For this review, take the finished solid that the model builds, in its own axes (mm). A direction names the side the tool comes from. Give positions to 0.01 mm unless a question says otherwise; leave off trailing zeros. Order: outer loops, then holes, each group sorted by start corner. A loop starts at its lowest first (then second) coordinate and runs counter-clockwise, first axis right, second up. Notation, with made-up numbers: (85.25, -28.75) - (133.25, -28.75) arc R23 cw to (133.25, -1.75) - close; hole circle Ø5 at (58, -16.75). An arc over 180 degrees is marked (long way). Use a Markdown table: item, result. Add a question column.
1) Machinability: for faces 4 (the face through (-242.37, -125.525, 1.479)), 5 (the face through (-214.32, -123.41, 1.48)), 6 (the face through (-24.751, -65.135, 1.479)), which of the approach directions +Z, -Z, +X, -X, +Y, -Y give a long, thin tool a straight path to every point of the face, cutting with its end or side? Answer none if there is none.
2) We need section C-C on y = -44.5. Write out the cut boundary in (x, z).
3) We need section B-B on z = 2.45. Give the number of separate pieces and of enclosed holes in the cut face, then the cut area to 3 significant figures.
4) Mouldability with a two-part tool opening along X and no side actions: class faces 1 (the face through (-270.05, -107.925, 1.479)), 2 (the face through (-117.616, -108.409, 1.479)), 3 (the face through (-169, -32, 3)) as released by +X, released by -X, zero draft, split by the parting line, or undercut.
5) Clearance check with flat-ended pins moving along their axes: P1, Ø1.5, axis at y = -16.5, z = 2.5, coming from the -X side; P2, Ø0.9, axis at x = -158.5, z = 2, coming from the +Y side; P3, Ø1.5, axis at y = -10.5, z = 2, coming from the -X side. State where each tip first meets the part, or that it passes through.
6) Wall thickness on L1, parallel to X at y = -106, z = 0.95; L2, parallel to X at y = -125, z = 1.9; L3, parallel to Y at x = -226.5, z = 2.65: over which ranges is each line inside the solid? List them lowest first.
7) We need section A-A on x = -33. Write out the cut boundary in (y, z), then the cut area to 3 significant figures.
```python
from build123d import *

# Parameters (mm, degrees)
BOSS_EXTRU_1_DEPTH = 3


with BuildPart() as part:
    # Esquisse1 → Boss.-Extru.1 (new body)
    with BuildSketch(Plane.XY):
        Polygon((-179.931816419, -11.401531345), (-180.017838024, -11.701531345), (-185.57619805, -31.086289447), (-167.791072806, -36.185021562), (-127.904950096, -24.747859919), (-17.351203316, 6.946262636), (-14.877374555, 5.574907028), (2.556514314, -55.224288823), (1.185265633, -57.698086926), (-51.424530344, -72.783703169), (-57.630729871, -89.716454796), (-63.024672228, -92.169507978), (-104.349665635, -118.563827288), (-107.470944884, -118.248029963), (-128.050089261, -98.290842938), (-133.151477342, -93.715936913), (-202.439042401, -93.715936913), (-207.540430482, -98.290842938), (-228.119574859, -118.248029963), (-231.240854108, -118.563827288), (-272.565847516, -92.169507978), (-277.959789872, -89.716454796), (-284.165989399, -72.783703169), (-336.775785376, -57.698086926), (-338.147034057, -55.224288823), (-320.713145188, 5.574907028), (-318.239316427, 6.946262636), (-207.685569647, -24.747859919), (-203.944682562, -11.701531345), (-203.858660957, -11.401531345), (-205.982988252, -11.401531345), (-221.327812729, -7.001473731), (-228.053301524, -5.072970852), (-324.305573392, 22.521130566), (-330.707501003, 18.97225141), (-353.72243999, -61.290379239), (-350.173829458, -67.692242105), (-294.328030452, -83.705767284), (-288.532091821, -99.519179156), (-251.042661762, -116.568594893), (-233.45174982, -134.735979634), (-226.135810249, -134.851076098), (-202.175390102, -111.650948678), (-133.415129641, -111.650948678), (-109.454709494, -134.851076098), (-102.138769923, -134.735979634), (-84.547857981, -116.568594893), (-47.058427922, -99.519179156), (-41.262489291, -83.705767284), (14.583309715, -67.692242105), (18.131920247, -61.290379239), (-4.88301874, 18.97225141), (-11.284946351, 22.521130566), (-107.537218219, -5.072970852), (-114.262707014, -7.001473731), (-123.876268292, -9.758118068), (-129.607531491, -11.401531345), (-167.175777529, -11.401531345), align=None)
        Polygon((-226.456549288, -126.726039887), (-228.072581173, -129.499661036), (-231.282623491, -129.486946945), (-232.876633924, -126.700611704), (-231.260602039, -123.926990555), (-228.050559721, -123.939704646), align=None, mode=Mode.SUBTRACT)
        Polygon((-201.720052379, -99.68218544), (-200.986265397, -102.807259839), (-203.325765724, -105.005275206), (-206.399053033, -104.078216174), (-207.132840016, -100.953141775), (-204.793339689, -98.755126408), align=None, mode=Mode.SUBTRACT)
        Polygon((-278.801584282, -92.701419409), (-279.761510176, -95.764600045), (-282.89426537, -96.464870154), (-285.067094671, -94.101959627), (-284.107168778, -91.03877899), (-280.974413583, -90.338508881), align=None, mode=Mode.SUBTRACT)
        Polygon((-341.674936445, -60.693756917), (-343.381773974, -63.412440235), (-346.589641557, -63.293617233), (-348.09067161, -60.456110913), (-346.38383408, -57.737427596), (-343.175966498, -57.856250598), align=None, mode=Mode.SUBTRACT)
        Polygon((-102.716844109, -126.851692582), (-104.440215275, -129.559925429), (-107.647299303, -129.421558643), (-109.131012166, -126.574959009), (-107.407640999, -123.866726161), (-104.200556971, -124.005092948), align=None, mode=Mode.SUBTRACT)
        Polygon((-129.102521286, -103.979530359), (-132.134816884, -105.032961295), (-134.563262635, -102.933631743), (-133.959412787, -99.780871255), (-130.927117189, -98.727440319), (-128.498671438, -100.826769871), align=None, mode=Mode.SUBTRACT)
        Polygon((-51.178552765, -91.36063702), (-50.649763202, -94.526851626), (-53.127390703, -96.567904124), (-56.133807767, -95.442742016), (-56.662597331, -92.27652741), (-54.18496983, -90.235474912), align=None, mode=Mode.SUBTRACT)
        Polygon((10.897318032, -57.794933915), (12.502351781, -60.574933915), (10.897318032, -63.354933915), (7.687250536, -63.354933915), (6.082216787, -60.574933915), (7.687250536, -57.794933915), align=None, mode=Mode.SUBTRACT)
        Polygon((-217.840116073, -13.876277124), (-214.696831686, -14.527657653), (-213.689301579, -17.575512049), (-215.825055858, -19.971985915), (-218.968340246, -19.320605385), (-219.975870353, -16.272750989), align=None, mode=Mode.SUBTRACT)
        Polygon((-326.25776259, 15.467139628), (-323.377643582, 16.884689567), (-320.709949819, 15.09920831), (-320.922375064, 11.896177113), (-323.802494072, 10.478627174), (-326.470187835, 12.264108431), align=None, mode=Mode.SUBTRACT)
        Polygon((-169.385770719, -24.817214521), (-166.175746894, -24.833958909), (-164.585236046, -27.622293282), (-166.204749024, -30.393883267), (-169.414772849, -30.37713888), (-171.005283697, -27.588804506), align=None, mode=Mode.SUBTRACT)
        Polygon((-117.981174931, -13.809459943), (-115.672169645, -16.039488624), (-116.448928491, -19.154160201), (-119.534692623, -20.038803095), (-121.84369791, -17.808774414), (-121.066939064, -14.694102838), align=None, mode=Mode.SUBTRACT)
        Polygon((-12.039253575, 16.891491339), (-9.240055353, 15.320178943), (-9.201252694, 12.110345974), (-11.961648258, 10.471825402), (-14.76084648, 12.043137798), (-14.799649138, 15.252970767), align=None, mode=Mode.SUBTRACT)
    extrude(amount=BOSS_EXTRU_1_DEPTH)


solid = part.part
```
Checked values:
| question | item | result |
|---|---|---|
| 1 | face 4 | +Z, -Z, -X, -Y |
| 1 | face 5 | +Z, -Z, -Y |
| 1 | face 6 | +Z, -Z |
| 2 | outline | (-348.91, 0) - (-335.07, 0) - (-335.07, 3) - (-348.91, 3) - close; (-0.52, 0) - (13.32, 0) - (13.32, 3) - (-0.52, 3) - close |
| 3 | separate pieces | 1 |
| 3 | enclosed holes | 13 |
| 3 | area | 11,900 mm² |
| 4 | face 1 | released by -X |
| 4 | face 2 | undercut |
| 4 | face 3 | zero draft |
| 5 | P1 | x = -341.09 |
| 5 | P2 | y = -11.4 |
| 5 | P3 | x = -339.37 |
| 6 | L1 | -274.28 to -250.91, -215.49 to -120.1, -84.68 to -61.31 |
| 6 | L2 | -242.88 to -231.89, -227.44 to -215.96, -119.63 to -108.13, -103.68 to -92.71 |
| 6 | L3 | -134.85 to -126.8, -126.65 to -116.68, -19.35 to -5.52 |
| 7 | outline | (-81.34, 0) - (-67.5, 0) - (-67.5, 3) - (-81.34, 3) - close; (2.46, 0) - (16.3, 0) - (16.3, 3) - (2.46, 3) - close |
| 7 | area | 83.0 mm² |
